from build123d import *

# Parameters (mm, degrees)
SKETCH2_R           = 1.5
SKETCH2_R_2         = 2.38125
BOSS_EXTRUDE1_DEPTH = 3.175
CHAMFER1_SIZE       = 1.27


with BuildPart() as part:
    # Sketch2 → Boss-Extrude1 (new body)
    with BuildSketch(Plane(origin=(0, 0, -51.1), x_dir=(-1, 0, 0), z_dir=(0, 0, -1))):
        Polygon((13.5, 388.72686963), (25.4, 388.72686963), (25.4, 343.22686963), (13.5, 343.22686963), (-13.5, 343.22686963), (-25.4, 343.22686963), (-25.4, 388.72686963), (-13.5, 388.72686963), align=None)
        with Locations(Location((10, 355.97686963, 0), (0, 0, 90))):
            Circle(SKETCH2_R, mode=Mode.SUBTRACT)
        with Locations(Location((10, 375.97686963, 0), (0, 0, 90))):
            Circle(SKETCH2_R, mode=Mode.SUBTRACT)
        with Locations(Location((-10, 375.97686963, 0), (0, 0, 90))):
            Circle(SKETCH2_R, mode=Mode.SUBTRACT)
        with Locations(Location((-10, 355.97686963, 0), (0, 0, 90))):
            Circle(SKETCH2_R, mode=Mode.SUBTRACT)
        with Locations(Location((19.45, 382.77686963, 0), (0, 0, 90))):
            Circle(SKETCH2_R_2, mode=Mode.SUBTRACT)
        with Locations(Location((-19.45, 382.77686963, 0), (0, 0, 270))):
            Circle(SKETCH2_R_2, mode=Mode.SUBTRACT)
        with Locations(Location((19.45, 349.17686963, 0), (0, 0, 270))):
            Circle(SKETCH2_R_2, mode=Mode.SUBTRACT)
        with Locations(Location((-19.45, 349.17686963, 0), (0, 0, 90))):
            Circle(SKETCH2_R_2, mode=Mode.SUBTRACT)
    extrude(amount=BOSS_EXTRUDE1_DEPTH)

    # Chamfer1
    chamfer1_edges = [part.edges().sort_by_distance(p)[0] for p in [
        (-10, 354.47686963, -54.275),
        (-10, 374.47686963, -54.275),
        (10, 374.47686963, -54.275),
        (10, 354.47686963, -54.275),
    ]]
    chamfer(chamfer1_edges, length=CHAMFER1_SIZE)


solid = part.part
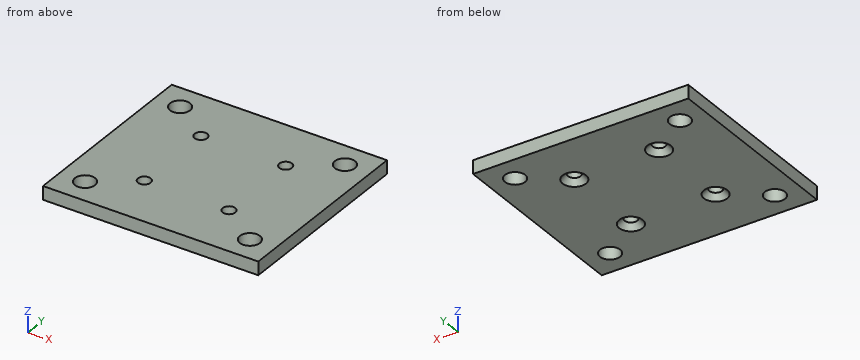
Read the model definition and answer for the solid it produces. Units are mm, in the model's axes. Give positions to 0.01 mm unless a question says otherwise; leave off trailing zeros. Write each loop counter-clockwise with the first axis right and the second up, starting at its lowest first coordinate (ties: lowest second). Pieces come first, ordered by that corner, then holes. Notation, with made-up numbers: M -30,45 L 4,45 A22 cw 4,73 Z; hole C 36.5,-28.5 d1. An arc over 180 degrees is marked long. One line per item, written item: value. Start each with the question number.
(1) Find section B-B (z = -51.8). Give the number of separate pieces and of enclosed holes in the cut face, plus the area to 3 significant figures.
(2) Find section A-A (x = -19.45). Determine the outline of the cut face in (y, z) (3 decimals).
(3) Find section C-C (x = 10). Determine the outline of the cut face in (y, z) (3 decimals).
(4) Find the intervals of material crossed by line 1 (X direction, y = 383, z = -52.9); line 2 (X direction, y = 355, z = -51.9); line 3 (Y direction, x = -11, z = -52.05), in increasing order.
(5) Flat-ended cylindrical pins translate along their axes: pin 1 Ø5 at (x, y) = (10, 355.98) entering from -Z; pin 2 Ø3.5 at (x, y) = (-10, 355.98) entering from -Z. Find the tip coordinate at first contact, or state that the pin passes through.
Results below:
1. separate pieces: 1
1. enclosed holes: 8
1. area: 2,210 mm^2
2. outline: M 343.227,-54.275 L 346.796,-54.275 L 346.796,-51.1 L 343.227,-51.1 Z; M 351.558,-54.275 L 380.396,-54.275 L 380.396,-51.1 L 351.558,-51.1 Z; M 385.158,-54.275 L 388.727,-54.275 L 388.727,-51.1 L 385.158,-51.1 Z
3. outline: M 343.227,-54.275 L 353.207,-54.275 L 354.477,-53.005 L 354.477,-51.1 L 343.227,-51.1 Z; M 357.477,-53.005 L 358.747,-54.275 L 373.207,-54.275 L 374.477,-53.005 L 374.477,-51.1 L 357.477,-51.1 Z; M 377.477,-53.005 L 378.747,-54.275 L 388.727,-54.275 L 388.727,-51.1 L 377.477,-51.1 Z
4. line 1: x = -25.4 to -21.82, -17.08 to 17.08, 21.82 to 25.4
4. line 2: x = -25.4 to -11.14, -8.86 to 8.86, 11.14 to 25.4
4. line 3: y = 343.23 to 354.86, 357.09 to 374.86, 377.09 to 388.73
5. pin 1: stops at z = -54.01
5. pin 2: stops at z = -53.26
